from build123d import *

# Parameters (mm, degrees)
SKETCH001_R          = 6.630792
SKETCH001_R_2        = 10.498697
PAD_DEPTH            = 40
POCKET_DEPTH         = 32
POCKET001_DEPTH      = 9
POCKET002_DEPTH      = 5
POCKET003_DEPTH      = 10
SKETCH005_W          = 94.298041
SKETCH005_H          = 32.366995
POCKET004_DEPTH      = 34.422931
POCKET004_DEPTH_BACK = -34.422931


with BuildPart() as part:
    # Sketch001 → Pad (new body)
    with BuildSketch(Plane.XY):
        with BuildLine():
            ThreePointArc((-19.821, 22.046589), (-32.196342, 34.421931), (-44.571684, 22.046589))
            Line((-44.571684, 22.046589), (-44.571684, -22.046589))
            ThreePointArc((-44.571684, -22.046589), (-32.196342, -34.421931), (-19.821, -22.046589))
            Line((-19.821, -22.046589), (-5.074877, -22.046589))
            Line((45.00301, -14.074842), (-5.074877, -22.046589))
            ThreePointArc((45.00301, -14.074842), (58.588852, 0.32742), (44.348215, 14.082584))
            Line((-4.908487, 22.046589), (44.348215, 14.082584))
            Line((-19.821, 22.046589), (-4.908487, 22.046589))
        make_face()
        with Locations((-32.196342, 22.046589)):
            Circle(SKETCH001_R, mode=Mode.SUBTRACT)
        with Locations((-32.196342, -22.046589)):
            Circle(SKETCH001_R, mode=Mode.SUBTRACT)
        with Locations((44.509155, 0)):
            Circle(SKETCH001_R_2, mode=Mode.SUBTRACT)
    extrude(amount=PAD_DEPTH)

    # Sketch002 → Pocket (cut)
    with BuildSketch(Plane.XY.offset(40)):
        with BuildLine():
            ThreePointArc((-19.354646, 22.067252), (-32.292828, 34.810367), (-45.101294, 21.936878))
            Line((-45.101294, 21.936878), (-45.101294, -21.936878))
            ThreePointArc((-45.101294, -21.936878), (-32.29321, -34.810365), (-19.354654, -22.068018))
            Line((-23.390144, -22.068018), (-19.354654, -22.068018))
            Line((-23.390144, -3.218184), (-23.390144, -22.068018))
            Line((-44.728828, -3.218184), (-23.390144, -3.218184))
            Line((-44.728828, 3.218184), (-44.728828, -3.218184))
            Line((-23.390144, 3.218184), (-44.728828, 3.218184))
            Line((-23.390144, 22.067252), (-23.390144, 3.218184))
            Line((-19.354646, 22.067252), (-23.390144, 22.067252))
        make_face()
    extrude(amount=-POCKET_DEPTH, mode=Mode.SUBTRACT)

    # Sketch003 (on Face17 of Pocket) → Pocket001 (cut)
    with BuildSketch(Plane.XZ.offset(3.218184)):
        Polygon((-22.446281, 41.467144), (-45.756935, 6.110793), (-48.87989, 41.467144), align=None)
    extrude(amount=-POCKET001_DEPTH, mode=Mode.SUBTRACT)

    # Sketch → Pocket002 (cut)
    with BuildSketch(Plane.XY.offset(40)):
        with BuildLine():
            Line((-51.758927, -23.019849), (-51.572633, 22.533843))
            Line((-51.572633, 22.533843), (-4.833725, 22.533843))
            Line((-4.833725, 22.533843), (44.348215, 14.082584))
            ThreePointArc((44.348215, 14.082584), (30.429458, -0.32742), (45.00301, -14.074842))
            Line((45.00301, -14.074842), (-5.186409, -23.019849))
            Line((-51.758927, -23.019849), (-5.186409, -23.019849))
        make_face()
    extrude(amount=-POCKET002_DEPTH, mode=Mode.SUBTRACT)

    # Sketch004 (on Face23 of Pocket002) → Pocket003 (cut)
    with BuildSketch(Plane.XZ.offset(3.218184)):
        Polygon((-20.760923, 38.424774), (-49.368839, 1.506935), (-41.058918, 38.424774), align=None)
    extrude(amount=-POCKET003_DEPTH, mode=Mode.SUBTRACT)

    # Sketch005 → Pocket004 (cut, two sides)
    with BuildSketch(Plane.XZ) as pocket004_sk:
        with Locations((37.4594, 9.552193)):
            Rectangle(SKETCH005_W, SKETCH005_H)
    extrude(amount=-POCKET004_DEPTH, mode=Mode.SUBTRACT)
    extrude(pocket004_sk.sketch, amount=-POCKET004_DEPTH_BACK, mode=Mode.SUBTRACT)


solid = part.part
For this review, take the finished solid that the model builds, in its own axes (mm). A direction names the side the tool comes from. Coordinates: 2 decimals unless noted, no trailing zeros. Order: outer loops, then holes, each group sorted by start corner. A loop starts at its lowest first (then second) coordinate and runs counter-clockwise, first axis right, second up. Notation, with made-up numbers: (33, 4) - (90, 4) arc R11 cw to (90, 25) - close; hole circle Ø5 at (-30.5, 31). An arc over 180 degrees is marked (long way). Use one line per item in the form item = value.
Q1. For P1, Ø20, axis at x = -30.5, y = 17, coming from the +Z side; P2, Ø10.5, axis at x = -34.5, z = 23, coming from the -Y side; P3, Ø20.5, axis at y = 8.5, z = 23.5, coming from the -X side; P4, Ø2, axis at y = 26, z = 9.5, coming from the -X side, all flat-tipped, find the tip position at first contact; note any pin that passes through.
Checked values:
P1 = 35
P2 = -3.22
P3 = -39.13
P4 = through
Q2. Consider section B-B (x = 38). Give the boundary of the cut face in (y, z), then the cut area to 3 significant figures.
Checked values:
outline = (-15.19, 25.74) - (-8.24, 25.74) - (-8.24, 40) - (-12.49, 40) - (-12.49, 35) - (-15.19, 35) - close; (8.24, 25.74) - (15.11, 25.74) - (15.11, 35) - (12.49, 35) - (12.49, 40) - (8.24, 40) - close
area = 171 mm2
Q3. For probe 1 along Z at (x, y) = (36.5, 11.5); probe 2 along Z at (x, y) = (-17, 0.5); probe 3 along X at (y, z) = (-14, 18.5), list the stretches that pass through material, from the lowest coordinate up. Write a range as from..to.
Checked values:
probe_1 = 25.74..40
probe_2 = 0..35
probe_3 = -23.39..-9.69
Q4. Consider section D-D (y = -25). Give the boundary of the cut face in (x, z), then the cut area to 3 significant figures.
Checked values:
outline = (-44.21, 0) - (-38.13, 0) - (-38.13, 8) - (-44.21, 8) - close; (-26.26, 0) - (-20.18, 0) - (-20.18, 8) - (-26.26, 8) - close
area = 97.3 mm2
Q5. Draft analysis for pull direction Y (two halves, no side actions). For faces 5 (the flat face through (16, 0, 25.736)), 6 (the cylindrical face through (-33.63, -28.52, 3.94)), 7 (the cylindrical face through (-32.29, -34.42, 3.16)), state which applies: +Y half, -Y half, draft (parallel to the pull), parting line (faces both ways), or undercut.
Checked values:
face_5 = draft
face_6 = undercut
face_7 = -Y half
Q6. Consider section A-A (y = 0). Give the boundary of the cut face in (x, z), then the cut area to 3 significant figures.
Checked values:
outline = (-44.57, 0) - (-9.69, 0) - (-9.69, 25.74) - (34.01, 25.74) - (34.01, 40) - (30.43, 40) - (30.43, 35) - (-23.41, 35) - (-44.57, 7.7) - close; (55.01, 25.74) - (58.59, 25.74) - (58.59, 40) - (55.01, 40) - close
area = 1,410 mm2
Q7. For faces 1 (the flat face through (-14, -22.047, 17)), 2 (the flat face through (-23.39, -13, 22)), 3 (the flat face through (-22, -22.068, 22)), 4 (the flat face through (-9.69, 0, 13)), list the 3-axis set-ups (+Z, -Z, +X, -X, +Y, -Y) from which the entire face can be reached by the end or side of a thin tool; tool diameter is ignored.
Checked values:
face_1 = +Z, -Z, +X, -Y
face_2 = +Z, -X, -Y
face_3 = +Z, +X, -X, -Y
face_4 = -Z, +X, +Y, -Y
